from build123d import *

# Parameters (mm, degrees)
SKETCH1_W           = 103
SKETCH1_H           = 69
BOSS_EXTRUDE1_DEPTH = 3
SKETCH2_W           = 81
SKETCH2_H           = 47
CUT_EXTRUDE1_DEPTH  = 3
CUT_EXTRUDE2_DEPTH  = 2
FILLET2_R           = 2.5
FILLET3_R           = 2.5
CHAMFER1_SIZE       = 0.5
CUT_EXTRUDE3_DEPTH  = 2
SKETCH5_W           = 10
SKETCH5_H           = 2.5
BOSS_EXTRUDE2_DEPTH = 5
SKETCH6_W           = 8
SKETCH6_H           = 5.75
BOSS_EXTRUDE3_DEPTH = 5


with BuildPart() as part:
    # Sketch1 → Boss-Extrude1 (new body)
    with BuildSketch(Plane.XY):
        with Locations((62.328366078, 28.443882797)):
            Rectangle(SKETCH1_W, SKETCH1_H)
    extrude(amount=BOSS_EXTRUDE1_DEPTH)

    # Sketch2 → Cut-Extrude1 (cut)
    with BuildSketch(Plane.XY.offset(3)):
        with Locations((62.328366078, 28.443882797)):
            Rectangle(SKETCH2_W, SKETCH2_H)
    extrude(amount=-CUT_EXTRUDE1_DEPTH, mode=Mode.SUBTRACT)

    # Sketch3 → Cut-Extrude2 (cut)
    with BuildSketch(Plane.XY.offset(3)):
        Polygon((13.078366078, 55.193882797), (106.578366078, 55.193882797), (106.578366078, 1.693882797), (13.078366078, 1.693882797), (13.078366078, 20.943882797), (11.578366078, 20.943882797), (11.578366078, 35.943882797), (13.078366078, 35.943882797), align=None)
    extrude(amount=-CUT_EXTRUDE2_DEPTH, mode=Mode.SUBTRACT)

    # Fillet2
    fillet2_edges = [part.edges().sort_by_distance(p)[0] for p in [
        (113.828366078, -6.056117203, 1.5),
        (10.828366078, -6.056117203, 1.5),
        (10.828366078, 62.943882797, 1.5),
        (113.828366078, 62.943882797, 1.5),
    ]]
    fillet(fillet2_edges, radius=FILLET2_R)

    # Fillet3
    fillet3_edges = [part.edges().sort_by_distance(p)[0] for p in [
        (21.828366078, 4.943882797, 0.5),
        (21.828366078, 51.943882797, 0.5),
        (102.828366078, 51.943882797, 0.5),
        (102.828366078, 4.943882797, 0.5),
    ]]
    fillet(fillet3_edges, radius=FILLET3_R)

    # Chamfer1
    chamfer1_edges = [part.edges().sort_by_distance(p)[0] for p in [
        (62.328366078, 4.943882797, 0),
        (102.828366078, 28.443882797, 0),
        (22.560599125, 51.21164975, 0),
        (22.560599125, 5.676115844, 0),
        (102.096133031, 5.676115844, 0),
        (102.096133031, 51.21164975, 0),
        (21.828366078, 28.443882797, 0),
        (62.328366078, 51.943882797, 0),
    ]]
    chamfer(chamfer1_edges, length=CHAMFER1_SIZE)

    # Sketch4 → Cut-Extrude3 (cut)
    with BuildSketch(Plane.XY.offset(3)):
        Polygon((16.828366078, 55.193882797), (16.828366078, 56.943882797), (12.828366078, 56.943882797), (12.828366078, 52.343882797), (13.078366078, 52.343882797), (13.078366078, 55.193882797), align=None)
        Polygon((103.828366078, 55.193882797), (103.828366078, 57.443882797), (108.828366078, 57.443882797), (108.828366078, 52.443882797), (106.578366078, 52.443882797), (106.578366078, 55.193882797), align=None)
        Polygon((16.828366078, 1.693882797), (16.828366078, -0.056117203), (12.828366078, -0.056117203), (12.828366078, 4.343882797), (13.078366078, 4.343882797), (13.078366078, 1.693882797), align=None)
        Polygon((103.828366078, 1.693882797), (103.828366078, -0.556117203), (108.828366078, -0.556117203), (108.828366078, 4.443882797), (106.578366078, 4.443882797), (106.578366078, 1.693882797), align=None)
    extrude(amount=-CUT_EXTRUDE3_DEPTH, mode=Mode.SUBTRACT)

    # Sketch5 → Boss-Extrude2 (add)
    with BuildSketch(Plane.XY.offset(3)):
        with Locations((84.328366078, 59.693882797)):
            Rectangle(SKETCH5_W, SKETCH5_H)
        with Locations((40.328366078, 59.693882797)):
            Rectangle(SKETCH5_W, SKETCH5_H)
    extrude(amount=BOSS_EXTRUDE2_DEPTH)

    # Sketch6 → Boss-Extrude3 (add)
    with BuildSketch(Plane.XY.offset(3)):
        with Locations((62.328366078, -1.181117203)):
            Rectangle(SKETCH6_W, SKETCH6_H)
    extrude(amount=BOSS_EXTRUDE3_DEPTH)


solid = part.part
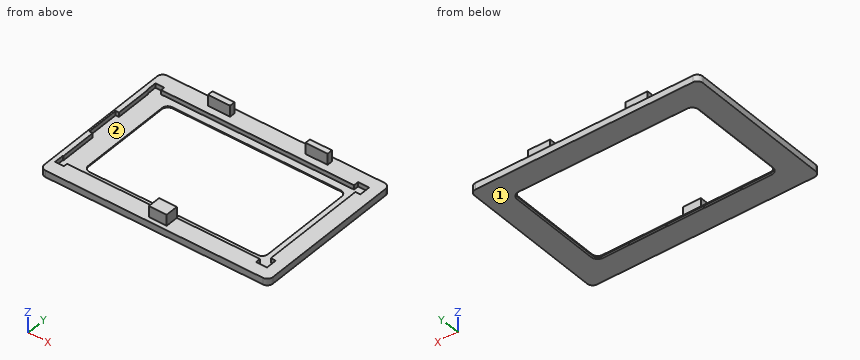
Part model, mm, in its own coordinate system. Face numbers are marked on the shaded views. Coordinates: 2 decimals unless noted, no trailing zeros. Order: outer loops, then holes, each group sorted by start corner. A loop starts at its lowest first (then second) coordinate and runs counter-clockwise, first axis right, second up. Notation, with made-up numbers: (45, 32) - (68, 32) arc R19 cw to (68, 64) - close; hole circle Ø8 at (66.25, 54.5). An arc over 180 degrees is marked (long way). Use CSV: the item, a comma, the result in double quotes.
Item 1: Drop flat-ended pins along their axis: P1, Ø0.8, axis at x = 12, z = 2.5, coming from the +Y side; P2, Ø4, axis at y = 48.5, z = 6.5, coming from the -X side; P3, Ø3, axis at y = 60.5, z = 6, coming from the -X side; P4, Ø4, axis at x = 83.5, z = 6.5, coming from the +Y side. Give the stop position or say it passes through.
Solved:
P1,"stops at y = 62.77"
P2,"passes through"
P3,"stops at x = 35.33"
P4,"stops at y = 60.94"
Item 2: Mould opens along Y. For the marked faces 1 and 2 say: +Y half, -Y half, draft (parallel to the pull), parting line (faces both ways), or undercut.
Solved:
face 1,"draft"
face 2,"undercut"
Item 3: Saw through at D-D on x = 73. Give the cut face in (y, z), and give its area (4 significant figures).
Solved:
outline,"(-6.06, 0) - (4.44, 0) - (4.94, 0.5) - (4.94, 1) - (1.69, 1) - (1.69, 3) - (-6.06, 3) - close; (51.94, 0.5) - (52.44, 0) - (62.94, 0) - (62.94, 3) - (55.19, 3) - (55.19, 1) - (51.94, 1) - close"
area,"52.75 mm²"
Item 4: Probe probe 1 along X at (y, z) = (38, 1.5); probe 2 along Y at (x, z) = (61.5, 2.5); probe 3 along Y at (x, z) = (105.5, 1.75). List the from-to ranges inside material, lowest first.
Solved:
probe 1,"x = 10.83 to 13.08, 106.58 to 113.83"
probe 2,"y = -6.06 to 1.69, 55.19 to 62.94"
probe 3,"y = -6.06 to -0.56, 57.44 to 62.94"
Item 5: Saw through at B-B on z = 6. Give the cut face in (x, y), and give its area (3 significant figures).
Solved:
outline,"(35.33, 58.44) - (45.33, 58.44) - (45.33, 60.94) - (35.33, 60.94) - close; (58.33, -4.06) - (66.33, -4.06) - (66.33, 1.69) - (58.33, 1.69) - close; (79.33, 58.44) - (89.33, 58.44) - (89.33, 60.94) - (79.33, 60.94) - close"
area,"96.0 mm²"
Item 6: Saw through at A-A on x = 60.5. Give the cut face in (y, z).
Solved:
outline,"(-6.06, 0) - (4.44, 0) - (4.94, 0.5) - (4.94, 1) - (1.69, 1) - (1.69, 8) - (-4.06, 8) - (-4.06, 3) - (-6.06, 3) - close; (51.94, 0.5) - (52.44, 0) - (62.94, 0) - (62.94, 3) - (55.19, 3) - (55.19, 1) - (51.94, 1) - close"
Item 7: Saw through at C-C on y = 26. Give the cut face in (x, z).
Solved:
outline,"(10.83, 0) - (21.33, 0) - (21.83, 0.5) - (21.83, 1) - (11.58, 1) - (11.58, 3) - (10.83, 3) - close; (102.83, 0.5) - (103.33, 0) - (113.83, 0) - (113.83, 3) - (106.58, 3) - (106.58, 1) - (102.83, 1) - close"
